Geometry: see drawing. Coordinates: mm, zero at the bounding-box minimum. A direction names the side the tool comes from. Give positions to 0.01 mm unless a question says otherwise; leave off trailing zeros. Write each loop counter-clockwise with the first axis right and the second up, starting at its lowest first coordinate (ties: lowest second). Pieces come first, ordered by that corner, then holes. Notation, with made-up numbers: (3.25, -22.75) -> (12.25, -22.75) arc R14 cw to (12.25, -2.75) -> close; hole circle Ø3 at (-12, -6.5). An arc over 180 degrees is marked (long way). Use CSV: the item, a comma, the result in double quotes. Start each with the question number.
1) Section D-D (z = 14.5). Output: boundary loops of the cut face in (x, y), plus the area to 3 significant figures.
2) Set-up query: the marked faces 5 and 6. Return all of +Z, -Z, +X, -X, +Y, -Y with unobstructed straight access to the full face (end or side cutting, diameter ignored); none if empty.
3) Section B-B (z = 5.25). Output: boundary loops of the cut face in (x, y).
4) Material intervals for line 1 (X direction, y = 1.75, z = 5.25); line 2 (X direction, y = 0.8, z = 15); line 3 (X direction, y = 1.9, z = 1), sorted ascending. Write a range as [from, to].
5) Contact query for flat-ended pins moving along their axis: P1, Ø1.6, axis at x = 1, y = 3.5, coming from the +Z side; P2, Ø1.5, axis at y = 4, z = 2, coming from the +X side. Output: stop coordinate, or through.
6) Draft query along X for the marked faces 1, 2, 3 and 4. Return one class per face: pulls with the +X half, pulls with the -X half, needs draft (parallel to the pull), parting line crosses it, or undercut.
7) Section C-C (y = 3.8). Output: boundary loops of the cut face in (x, z), plus the area to 3 significant figures.
8) Section A-A (x = 8.25). Output: boundary loops of the cut face in (y, z).
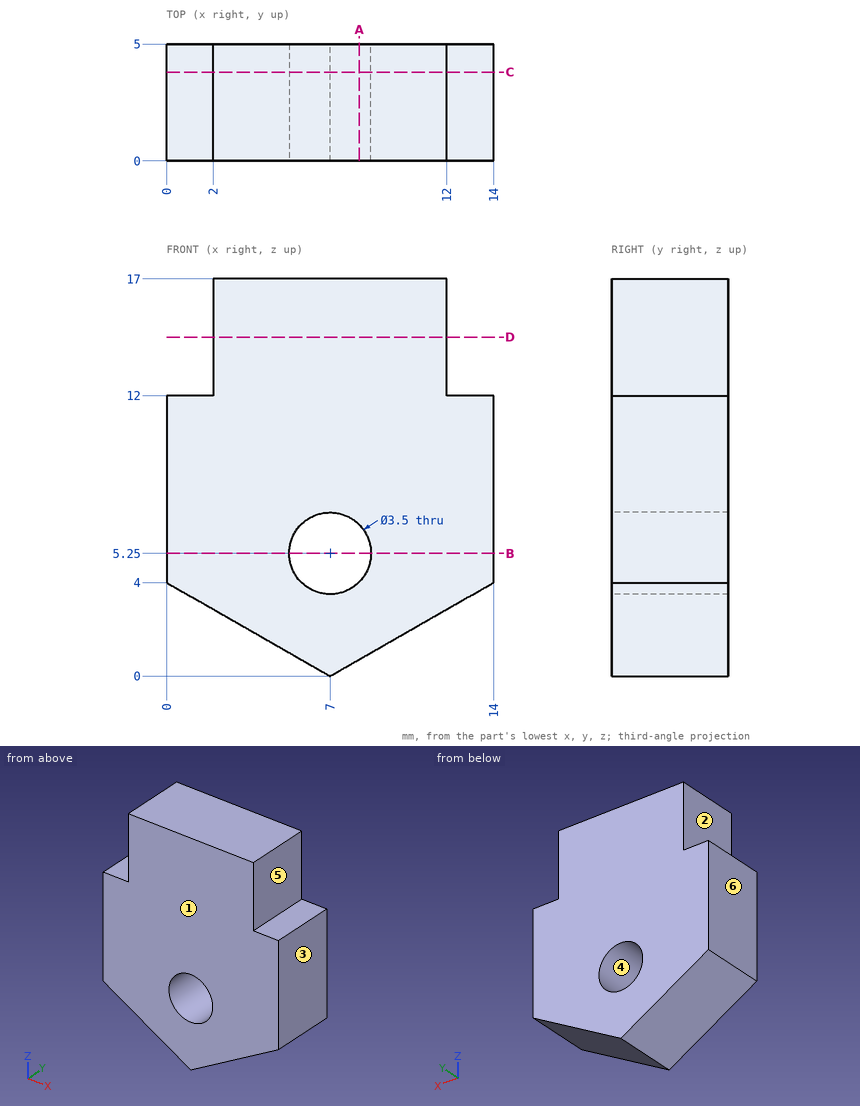
Answers follow:
1,outline,"(2, 0) -> (12, 0) -> (12, 5) -> (2, 5) -> close"
1,area,"50.0 mm^2"
2,face 5,"+Z, +X, +Y, -Y"
2,face 6,"+Z, -Z, -X, +Y, -Y"
3,outline,"(0, 0) -> (5.25, 0) -> (5.25, 5) -> (0, 5) -> close; (8.75, 0) -> (14, 0) -> (14, 5) -> (8.75, 5) -> close"
4,line 1,"x = [0, 5.25], [8.75, 14]"
4,line 2,"x = [2, 12]"
4,line 3,"x = [5.25, 8.75]"
5,P1,"stops at z = 12"
5,P2,"stops at x = 11.81"
6,face 1,"needs draft"
6,face 2,"pulls with the -X half"
6,face 3,"pulls with the +X half"
6,face 4,"undercut"
7,outline,"(0, 4) -> (7, 0) -> (14, 4) -> (14, 12) -> (12, 12) -> (12, 17) -> (2, 17) -> (2, 12) -> (0, 12) -> close; hole circle Ø3.5 at (7, 5.25)"
7,area,"180 mm^2"
8,outline,"(0, 0.71) -> (5, 0.71) -> (5, 4.03) -> (0, 4.03) -> close; (0, 6.47) -> (5, 6.47) -> (5, 17) -> (0, 17) -> close"
